Could you check a few things on this model? Use its own coordinates, in mm. A direction names the side the tool comes from. Round coordinates to 2 decimals unless told otherwise and drop trailing zeros. Write each loop counter-clockwise with the first axis right and the second up, starting at its lowest first coordinate (ties: lowest second). Pieces come first, ordered by that corner, then holes. Notation, with made-up numbers: (7.5, 55.5) -> (66.5, 55.5) arc R19 ccw to (66.5, 61.5) -> close; hole circle Ø11 at (26, 42). An arc over 180 degrees is marked (long way). Answer in a Markdown table with one row per item.
Autodesk Inventor part; units mm, degrees
ref_plane "Work Plane1" through (0, 0, 5.75) normal (0, 0, 1) x (1, 0, 0)
ref_plane "YZ Plane" through (0, 0, 0) normal (1, 0, 0) x (0, 1, 0)
ref_plane "XZ Plane" through (0, 0, 0) normal (0, 1, 0) x (-1, 0, 0)
sketch "Sketch1" plane through (0, 0, 0) normal (0, 1, 0) x (-1, 0, 0)
  circle A0 centre (0, 0) radius 5.75
  dimension "d0" = 11.5
extrude "Extrusion1" add sketch "Sketch1" along normal blind 155
sketch "Sketch2" plane through (0, 155, 0) normal (0, 1, 0) x (1, 0, 0)
  circle A0 centre (0, 0) radius 16
  dimension "d3" = 32
extrude "Extrusion2" add sketch "Sketch2" along normal blind 5
sketch "Sketch3" plane through (0, 160, 0) normal (0, 1, 0) x (1, 0, 0)
  circle A0 centre (0, 0) radius 9
  dimension "d6" = 18
extrude "Extrusion3" cut sketch "Sketch3" against normal blind 1
ref_plane "Work Plane1" through (0, 0, 5.75) normal (0, 0, 1) x (1, 0, 0)
sketch "Sketch4" plane through (0, 0, 5.75) normal (0, 0, 1) x (1, 0, 0)
  line L0 (5.75, 155) -> (-5.75, 155)
  line L1 (5.75, 0) -> (-5.75, 0)
  line L2 (0, 0) -> (0, 5)
  circle A0 centre (0, 5) radius 1.5
  dimension "d9" = 5
  dimension "d10" = 3
extrude "Extrusion4" cut sketch "Sketch4" against normal blind 11.5
chamfer "Chamfer1" distance 1 angle 45 1 edges at (5.75, 0, 0)
sketch "Sketch5" plane through (0, 0, 0) normal (0, 0, 1) x (1, 0, 0)
  line L0 (0, 0) -> (0, 42.5)
  line L1 (0, 42.5) -> (0, 32.5)
  line L2 (0, 42.5) -> (0, 52.5)
  circle A0 centre (0, 52.5) radius 2.5
  dimension "d16" = 42.5
  dimension "d17" = 10
  dimension "d18" = 10
  dimension "d19" = 5
extrude "Extrusion5" cut sketch "Sketch5" along normal mid plane 13
sketch "Sketch6" plane through (0, 160, 0) normal (0, 1, 0) x (1, 0, 0)
  circle A0 centre (0, 0) radius 16
  line L0 (-16, 0) -> (-9, 0)
  circle A1 centre (0, 0) radius 9
  circle A2 centre (-12.5, 0) radius 1.55
  dimension "d22" = 3.1
extrude "Extrusion6" cut sketch "Sketch6" against normal up to surface (5 mm away) contours A2 L0 | L0 A2
chamfer "Chamfer2" distance 0.3 angle 45 1 edges at (-14.05, 155, 0)
chamfer "Chamfer3" distance 0.3 angle 45 2 edges at (-2.5, 52.5, 5.1781) (-2.5, 52.5, -5.1781)
properties part number "wał_hamulca_dlugi" material "ABS Plastic"
1) Imagine slicing it at D-D, the plane z = -12. Please give me the cut outline in (x, y).
Findings:
| item | result |
|---|---|
| outline | (-10.58, 155) -> (10.58, 155) -> (10.58, 160) -> (-10.58, 160) -> close |
2) Imagine slicing it at A-A, the plane z = 0. Please give me the cut outline in (x, y).
Findings:
| item | result |
|---|---|
| outline | (-16, 155) -> (-14.35, 155) -> (-14.05, 155.3) -> (-14.05, 160) -> (-16, 160) -> close; (-10.95, 155.3) -> (-10.65, 155) -> (-5.75, 155) -> (-5.75, 1) -> (-4.75, 0) -> (4.75, 0) -> (5.75, 1) -> (5.75, 155) -> (16, 155) -> (16, 160) -> (9, 160) -> (9, 159) -> (-9, 159) -> (-9, 160) -> (-10.95, 160) -> close; hole circle Ø5 at (0, 52.5); hole circle Ø3 at (0, 5) |
3) Imagine slicing it at B-B, the plane x = -12.5. Please give me the cut outline in (y, z).
Findings:
| item | result |
|---|---|
| outline | (155, -9.99) -> (160, -9.99) -> (160, -1.55) -> (155.3, -1.55) -> (155, -1.85) -> close; (155, 1.85) -> (155.3, 1.55) -> (160, 1.55) -> (160, 9.99) -> (155, 9.99) -> close |
4) Thinking about a two-plate mould opening in X: for faces 1 (the face through (-1.172, 159.507, -8.923)), 2 (the face through (0, 0, 0)), 3 (the face through (0.75, 76.92, -5.7)), which applies, +X half, -X half, draft (parallel to the pull), parting line (faces both ways), or undercut?
Findings:
| item | result |
|---|---|
| face 1 | undercut |
| face 2 | draft |
| face 3 | parting line |
5) For faces 4 (the face through (-13.73, 157.68, 0.94)), 5 (the face through (0, 159, 0)), 6 (the face through (7, 155, 0)), which set-ups out of +Z, -Z, +X, -X, +Y, -Y let a thin tool reach every point of the face, with its end or its side?
Findings:
| item | result |
|---|---|
| face 4 | +Y, -Y |
| face 5 | +Y |
| face 6 | -Y |
6) Please list where these lines run through material, in increasing order: line 1 (X direction, y = 159.3, z = 0); line 2 (Y direction, x = 0, z = 3); line 3 (Z direction, x = 0, y = 159.5).
Findings:
| item | result |
|---|---|
| line 1 | x = -16 to -14.05, -10.95 to -9, 9 to 16 |
| line 2 | y = 0 to 3.5, 6.5 to 50, 55 to 159 |
| line 3 | z = -16 to -9, 9 to 16 |
7) For pin 1 (10 mm diameter, centred on y = 93, z = 0, fed in from +X); pin 2 (8 mm diameter, centred on x = -12.5, y = 110, fed in from -Z); pin 3 (2 mm diameter, centred on y = 67.5, z = 1, fed in from -X); pin 4 (2 mm diameter, centred on y = 115, z = 4.5, fed in from -X), each with a flat end and sliding along its axis, tell me the tip position at first contact or that it passes through.
Findings:
| item | result |
|---|---|
| pin 1 | stops at x = 5.75 |
| pin 2 | passes through |
| pin 3 | stops at x = -5.75 |
| pin 4 | stops at x = -4.56 |
8) Imagine slicing it at C-C, the plane y = 10.5. Please give me the cut outline in (x, z).
Findings:
| item | result |
|---|---|
| outline | circle Ø11.5 at (0, 0) |
